Geometry: see drawing. Coordinates: mm, zero at the bounding-box minimum. A direction names the side the tool comes from. Round coordinates to 2 decimals unless told otherwise and drop trailing zeros. Write each loop counter-clockwise with the first axis right and the second up, starting at its lowest first coordinate (ties: lowest second). Pieces come first, ordered by that corner, then holes. Notation, with made-up numbers: (-10, 84) - (21, 84) arc R21 ccw to (21, 91) - close; hole circle Ø6 at (13.5, 22.5). An arc over 180 degrees is marked (long way). One line per item, written item: value. Start each with the question number.
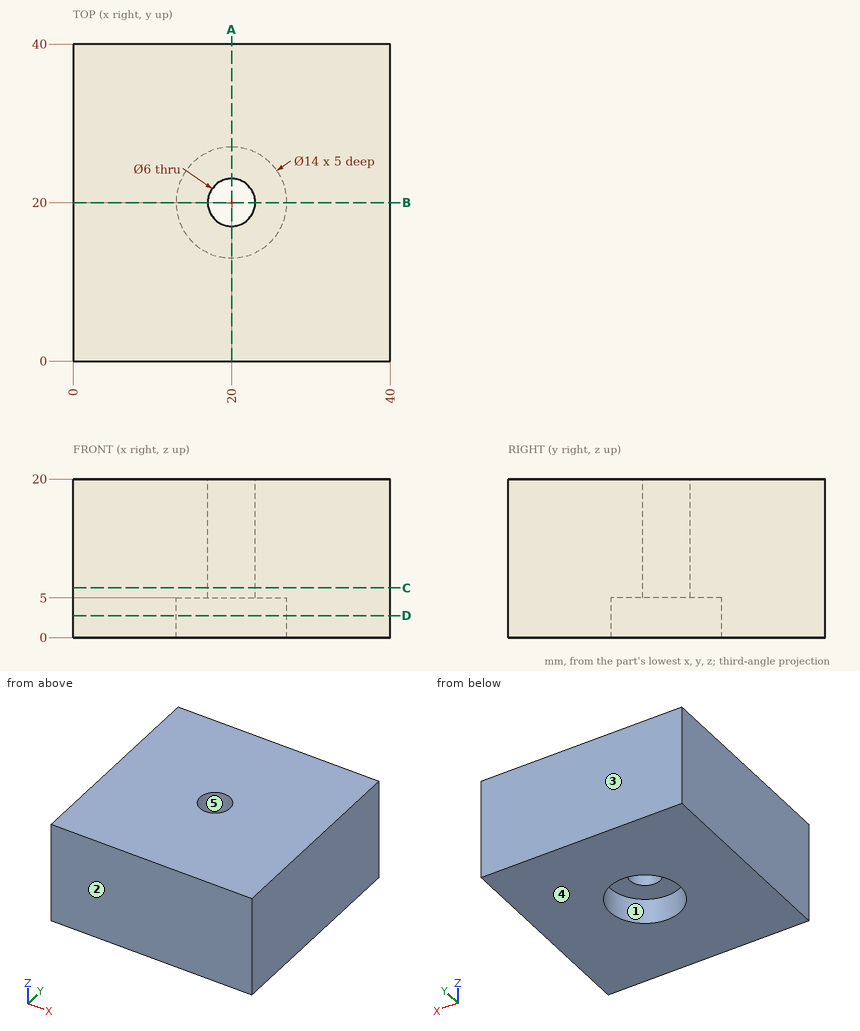
Q1. Cut plane D-D, the plane z = 2.75. Output: boundary loops of the cut face in (x, y), and give its area (3 significant figures).
Q2. Contact query for a flat-ended pin moving along its axis: pin 1 Ø4 at (x, y) = (20.5, 17) entering from -Z. Output: stop coordinate, or through.
Q3. Cut plane A-A, the plane x = 20. Output: boundary loops of the cut face in (y, z), and give its area (3 significant figures).
Q4. Material intervals for probe 1 along X at (y, z) = (20, 3.6); probe 2 along Y at (x, z) = (20, 6), sorted ascending. Write a range as from..to.
Q5. Access query for the marked faces 1 and 2. Directions: +Z, -Z, +X, -X, +Y, -Y. A direction counts if a zero-diameter tool reaches every point of the face in a straight line with its end or side. Return the directions, or none.
Q6. Cut plane C-C, the plane z = 6.25. Output: boundary loops of the cut face in (x, y).
Q7. Pull-direction query (Y, two-part tool) for the marked faces 3, 4 and 5; classes: pulls with the +Y half, pulls with the -Y half, needs draft (parallel to the pull), parting line crosses it, or undercut.
A:
1. outline: (0, 0) - (40, 0) - (40, 40) - (0, 40) - close; hole circle Ø14 at (20, 20)
1. area: 1,450 mm²
2. pin 1: stops at z = 5
3. outline: (0, 0) - (13, 0) - (13, 5) - (17, 5) - (17, 20) - (0, 20) - close; (23, 5) - (27, 5) - (27, 0) - (40, 0) - (40, 20) - (23, 20) - close
3. area: 640 mm²
4. probe 1: x = 0..13, 27..40
4. probe 2: y = 0..17, 23..40
5. face 1: -Z
5. face 2: +Z, -Z, +X, -X, -Y
6. outline: (0, 0) - (40, 0) - (40, 40) - (0, 40) - close; hole circle Ø6 at (20, 20)
7. face 3: pulls with the +Y half
7. face 4: needs draft
7. face 5: undercut
